Work out the finished part from the listing and answer in its coordinate system (mm). A direction names the side the tool comes from. Round coordinates to 2 decimals unless told otherwise and drop trailing zeros. Write each loop counter-clockwise with the first axis right and the second up, starting at its lowest first coordinate (ties: lowest second). Pieces come first, ordered by that corner, then holes. Notation, with made-up numbers: M 53,-37.5 L 112,-37.5 A25 cw 112,-3.5 Z; hole C 69,4 d8. An arc over 180 degrees is marked long. Answer in a Markdown table with one row per item.
```python
from build123d import *

# Parameters (mm, degrees)
SKETCH1_R           = 6
BOSS_EXTRUDE1_DEPTH = 3
CUT_EXTRUDE4_DEPTH  = 10
BOSS_EXTRUDE2_DEPTH = 5
SKETCH3_R           = 4.5
BOSS_EXTRUDE3_DEPTH = 1
SKETCH4_R           = 3
CUT_EXTRUDE1_DEPTH  = 2
SKETCH5_R           = 1.5
CUT_EXTRUDE2_DEPTH  = 48.699580711
SKETCH6_R           = 1
CUT_EXTRUDE3_DEPTH  = 10
SKETCH8_R           = 1.5
CUT_EXTRUDE5_DEPTH  = 2
SKETCH9_R           = 1
CUT_EXTRUDE6_DEPTH  = 10


with BuildPart() as part:
    # Sketch1 → Boss-Extrude1 (new body)
    with BuildSketch(Plane(origin=(0, 0, 0), x_dir=(1, 0, 0), z_dir=(0, 1, 0))):
        with Locations(Location((0, 0, 0), (0, 0, 270))):
            Circle(SKETCH1_R)
    extrude(amount=BOSS_EXTRUDE1_DEPTH)

    # Sketch7 → Cut-Extrude4 (cut, through all)
    with BuildSketch(Plane.XZ):
        with BuildLine():
            Line((0.7, 3.684087404), (0, 3.05))
            Line((0, 3.05), (-0.7, 3.684087404))
            ThreePointArc((-0.7, 3.684087404), (-0.779668841, 3.668053503), (-0.858971523, 3.650296964))
            Line((-0.858971523, 3.650296964), (-1.240546761, 2.786313646))
            Line((-1.240546761, 2.786313646), (-2.137935164, 3.080865663))
            ThreePointArc((-2.137935164, 3.080865663), (-2.204194696, 3.033813729), (-2.269419066, 2.985337016))
            Line((-2.269419066, 2.985337016), (-2.266591718, 2.040848349))
            Line((-2.266591718, 2.040848349), (-3.206201915, 1.944934261))
            ThreePointArc((-3.206201915, 1.944934261), (-3.247595264, 1.875), (-3.287463436, 1.804185178))
            Line((-3.287463436, 1.804185178), (-2.900722375, 0.942501833))
            Line((-2.900722375, 0.942501833), (-3.720087228, 0.472706055))
            ThreePointArc((-3.720087228, 0.472706055), (-3.729457108, 0.391981737), (-3.737075512, 0.311073332))
            Line((-3.737075512, 0.311073332), (-3.033291781, -0.318811813))
            Line((-3.033291781, -0.318811813), (-3.590735663, -1.081257322))
            ThreePointArc((-3.590735663, -1.081257322), (-3.566461936, -1.158813729), (-3.540513282, -1.235825919))
            Line((-3.540513282, -1.235825919), (-2.641377482, -1.525))
            Line((-2.641377482, -1.525), (-2.840513282, -2.448261485))
            ThreePointArc((-2.840513282, -2.448261485), (-2.786793096, -2.509239774), (-2.73176414, -2.569039642))
            Line((-2.73176414, -2.569039642), (-1.792745019, -2.467501833))
            Line((-1.792745019, -2.467501833), (-1.599140348, -3.391938995))
            ThreePointArc((-1.599140348, -3.391938995), (-1.525262412, -3.425795466), (-1.450668162, -3.458043072))
            Line((-1.450668162, -3.458043072), (-0.634130657, -2.983350182))
            Line((-0.634130657, -2.983350182), (-0.081261521, -3.749119439))
            ThreePointArc((-0.081261521, -3.749119439), (0, -3.75), (0.081261521, -3.749119439))
            Line((0.081261521, -3.749119439), (0.634130657, -2.983350182))
            Line((0.634130657, -2.983350182), (1.450668162, -3.458043072))
            ThreePointArc((1.450668162, -3.458043072), (1.525262412, -3.425795466), (1.599140348, -3.391938995))
            Line((1.599140348, -3.391938995), (1.792745019, -2.467501833))
            Line((1.792745019, -2.467501833), (2.73176414, -2.569039642))
            ThreePointArc((2.73176414, -2.569039642), (2.786793096, -2.509239774), (2.840513282, -2.448261485))
            Line((2.840513282, -2.448261485), (2.641377482, -1.525))
            Line((2.641377482, -1.525), (3.540513282, -1.235825919))
            ThreePointArc((3.540513282, -1.235825919), (3.566461936, -1.158813729), (3.590735663, -1.081257322))
            Line((3.590735663, -1.081257322), (3.033291781, -0.318811813))
            Line((3.033291781, -0.318811813), (3.737075512, 0.311073332))
            ThreePointArc((3.737075512, 0.311073332), (3.729457108, 0.391981737), (3.720087228, 0.472706055))
            Line((3.720087228, 0.472706055), (2.900722375, 0.942501833))
            Line((2.900722375, 0.942501833), (3.287463436, 1.804185178))
            ThreePointArc((3.287463436, 1.804185178), (3.247595264, 1.875), (3.206201915, 1.944934261))
            Line((3.206201915, 1.944934261), (2.266591718, 2.040848349))
            Line((2.266591718, 2.040848349), (2.269419066, 2.985337016))
            ThreePointArc((2.269419066, 2.985337016), (2.204194696, 3.033813729), (2.137935164, 3.080865663))
            Line((2.137935164, 3.080865663), (1.240546761, 2.786313646))
            Line((1.240546761, 2.786313646), (0.858971523, 3.650296964))
            ThreePointArc((0.858971523, 3.650296964), (0.779668841, 3.668053503), (0.7, 3.684087404))
        make_face()
    extrude(amount=-CUT_EXTRUDE4_DEPTH, mode=Mode.SUBTRACT)

    # Sketch2 → Boss-Extrude2 (add)
    with BuildSketch(Plane(origin=(0, 3, 0), x_dir=(1, 0, 0), z_dir=(0, 1, 0))):
        with BuildLine():
            Line((8, 0), (3.5, -43))
            ThreePointArc((3.5, -43), (0, -46.5), (-3.5, -43))
            Line((-3.5, -43), (-8, 0))
            ThreePointArc((-8, 0), (0, 8), (8, 0))
        make_face()
    extrude(amount=BOSS_EXTRUDE2_DEPTH)

    # Sketch3 → Boss-Extrude3 (add)
    with BuildSketch(Plane(origin=(0, 8, 0), x_dir=(1, 0, 0), z_dir=(0, 1, 0))):
        with Locations(Location((0, 0, 0), (0, 0, 270))):
            Circle(SKETCH3_R)
    extrude(amount=BOSS_EXTRUDE3_DEPTH)

    # Sketch4 → Cut-Extrude1 (cut)
    with BuildSketch(Plane(origin=(0, 9, 0), x_dir=(1, 0, 0), z_dir=(0, 1, 0))):
        with Locations(Location((0, 0, 0), (0, 0, 270))):
            Circle(SKETCH4_R)
    extrude(amount=-CUT_EXTRUDE1_DEPTH, mode=Mode.SUBTRACT)

    # Sketch5 → Cut-Extrude2 (cut, through all)
    with BuildSketch(Plane(origin=(0, 7, 0), x_dir=(1, 0, 0), z_dir=(0, 1, 0))):
        with Locations(Location((0, 0, 0), (0, 0, 270))):
            Circle(SKETCH5_R)
    extrude(amount=-CUT_EXTRUDE2_DEPTH, mode=Mode.SUBTRACT)

    # Sketch6 → Cut-Extrude3 (cut)
    with BuildSketch(Plane(origin=(0, 8, 0), x_dir=(1, 0, 0), z_dir=(0, 1, 0))):
        with Locations(Location((0, -13, 0), (0, 0, 270))):
            Circle(SKETCH6_R)
        with Locations(Location((0, -18, 0), (0, 0, 270))):
            Circle(SKETCH6_R)
        with Locations(Location((0, -23, 0), (0, 0, 270))):
            Circle(SKETCH6_R)
        with Locations(Location((0, -28, 0), (0, 0, 270))):
            Circle(SKETCH6_R)
        with Locations(Location((0, -33, 0), (0, 0, 270))):
            Circle(SKETCH6_R)
        with Locations(Location((0, -38, 0), (0, 0, 270))):
            Circle(SKETCH6_R)
        with Locations(Location((0, -43, 0), (0, 0, 270))):
            Circle(SKETCH6_R)
    extrude(amount=-CUT_EXTRUDE3_DEPTH, mode=Mode.SUBTRACT)

    # Sketch8 → Cut-Extrude5 (cut)
    with BuildSketch(Plane.XZ.offset(-3)):
        with BuildLine():
            Line((-0.858971523, 3.650296964), (-1.240546761, 2.786313646))
            Line((-1.240546761, 2.786313646), (-2.137935164, 3.080865663))
            ThreePointArc((-2.137935164, 3.080865663), (-2.204194696, 3.033813729), (-2.269419066, 2.985337016))
            Line((-2.269419066, 2.985337016), (-2.266591718, 2.040848349))
            Line((-2.266591718, 2.040848349), (-3.206201915, 1.944934261))
            ThreePointArc((-3.206201915, 1.944934261), (-3.247595264, 1.875), (-3.287463436, 1.804185178))
            Line((-3.287463436, 1.804185178), (-2.900722375, 0.942501833))
            Line((-2.900722375, 0.942501833), (-3.720087228, 0.472706055))
            ThreePointArc((-3.720087228, 0.472706055), (-3.729457108, 0.391981737), (-3.737075512, 0.311073332))
            Line((-3.737075512, 0.311073332), (-3.033291781, -0.318811813))
            Line((-3.033291781, -0.318811813), (-3.590735663, -1.081257322))
            ThreePointArc((-3.590735663, -1.081257322), (-3.566461936, -1.158813729), (-3.540513282, -1.235825919))
            Line((-3.540513282, -1.235825919), (-2.641377482, -1.525))
            Line((-2.641377482, -1.525), (-2.840513282, -2.448261485))
            ThreePointArc((-2.840513282, -2.448261485), (-2.786793096, -2.509239774), (-2.73176414, -2.569039642))
            Line((-2.73176414, -2.569039642), (-1.792745019, -2.467501833))
            Line((-1.792745019, -2.467501833), (-1.599140348, -3.391938995))
            ThreePointArc((-1.599140348, -3.391938995), (-1.525262412, -3.425795466), (-1.450668162, -3.458043072))
            Line((-1.450668162, -3.458043072), (-0.634130657, -2.983350182))
            Line((-0.634130657, -2.983350182), (-0.081261521, -3.749119439))
            ThreePointArc((-0.081261521, -3.749119439), (0, -3.75), (0.081261521, -3.749119439))
            Line((0.081261521, -3.749119439), (0.634130657, -2.983350182))
            Line((0.634130657, -2.983350182), (1.450668162, -3.458043072))
            ThreePointArc((1.450668162, -3.458043072), (1.525262412, -3.425795466), (1.599140348, -3.391938995))
            Line((1.599140348, -3.391938995), (1.792745019, -2.467501833))
            Line((1.792745019, -2.467501833), (2.73176414, -2.569039642))
            ThreePointArc((2.73176414, -2.569039642), (2.786793096, -2.509239774), (2.840513282, -2.448261485))
            Line((2.840513282, -2.448261485), (2.641377482, -1.525))
            Line((2.641377482, -1.525), (3.540513282, -1.235825919))
            ThreePointArc((3.540513282, -1.235825919), (3.566461936, -1.158813729), (3.590735663, -1.081257322))
            Line((3.590735663, -1.081257322), (3.033291781, -0.318811813))
            Line((3.033291781, -0.318811813), (3.737075512, 0.311073332))
            ThreePointArc((3.737075512, 0.311073332), (3.729457108, 0.391981737), (3.720087228, 0.472706055))
            Line((3.720087228, 0.472706055), (2.900722375, 0.942501833))
            Line((2.900722375, 0.942501833), (3.287463436, 1.804185178))
            ThreePointArc((3.287463436, 1.804185178), (3.247595264, 1.875), (3.206201915, 1.944934261))
            Line((3.206201915, 1.944934261), (2.266591718, 2.040848349))
            Line((2.266591718, 2.040848349), (2.269419066, 2.985337016))
            ThreePointArc((2.269419066, 2.985337016), (2.204194696, 3.033813729), (2.137935164, 3.080865663))
            Line((2.137935164, 3.080865663), (1.240546761, 2.786313646))
            Line((1.240546761, 2.786313646), (0.858971523, 3.650296964))
            ThreePointArc((0.858971523, 3.650296964), (0.779668841, 3.668053503), (0.7, 3.684087404))
            Line((0.7, 3.684087404), (0, 3.05))
            Line((0, 3.05), (-0.7, 3.684087404))
            ThreePointArc((-0.7, 3.684087404), (-0.779668841, 3.668053503), (-0.858971523, 3.650296964))
        make_face()
        with Locations(Location((0, 0, 0), (0, 0, 90))):
            Circle(SKETCH8_R, mode=Mode.SUBTRACT)
    extrude(amount=-CUT_EXTRUDE5_DEPTH, mode=Mode.SUBTRACT)

    # Sketch9 → Cut-Extrude6 (cut)
    with BuildSketch(Plane(origin=(0, 8, 0), x_dir=(1, 0, 0), z_dir=(0, 1, 0))):
        with BuildLine():
            ThreePointArc((-0.999557496, -32.970254191), (-3.566749104, -31.602893663), (-4.959923611, -29.049618831))
            Line((-4.959923611, -29.049618831), (-3.5, -43))
            ThreePointArc((-3.5, -43), (0, -46.5), (3.5, -43))
            Line((3.5, -43), (4.959923611, -29.049618831))
            ThreePointArc((4.959923611, -29.049618831), (3.566749104, -31.602893663), (0.999557496, -32.970254191))
            ThreePointArc((0.999557496, -32.970254191), (0.999889368, -32.98512545), (1, -33))
            ThreePointArc((1, -33), (-0.01487455, -33.999889368), (-0.999557496, -32.970254191))
        make_face()
        with Locations((0, -43)):
            Circle(SKETCH9_R, mode=Mode.SUBTRACT)
        with Locations((0, -38)):
            Circle(SKETCH9_R, mode=Mode.SUBTRACT)
    extrude(amount=-CUT_EXTRUDE6_DEPTH, mode=Mode.SUBTRACT)


solid = part.part
```
1. A tool of negligible diameter and unlimited length cuts with its end or side. For faces 1 (the flat face through (-1.3, 7, 1.3)), 2 (the flat face through (-2.73, 2.465, 1.994)), 3 (the cylindrical face through (0, 6, 14)), from which of +Z, -Z, +X, -X, +Y, -Y can it reach the whole face along a straight path? Write none if from no direction.
Calculated:
| item | result |
|---|---|
| face 1 | +Y |
| face 2 | -Y |
| face 3 | +Y, -Y |
2. Determine the mould class of faces 4 (the cylindrical face through (-3.54, 5.54, 31.63)), 5 (the flat face through (-3, 9, 1)), 6 (the flat face through (1.695, 2.465, -2.936)) for opening direction X: released by +X, released by -X, zero draft, split by the parting line, or undercut.
Calculated:
| item | result |
|---|---|
| face 4 | released by -X |
| face 5 | zero draft |
| face 6 | undercut |
3. The part is cut by section B-B (z = 23). Determine the outline of the cut face in (x, y), plus the area to 3 significant figures.
Calculated:
| item | result |
|---|---|
| outline | M -5.59,3 L -1,3 L -1,8 L -5.59,8 Z; M 1,3 L 5.59,3 L 5.59,8 L 1,8 Z |
| area | 45.9 mm² |
4. Consider line 1 along X through (y, z) = (6.55, 0); line 2 along Y through (x, z) = (0.25, 31); line 3 along Y through (x, z) = (-1.5, 4.5). Determine where each line is inside the solid, lowest interval first. Write a range as from..to.
Calculated:
| item | result |
|---|---|
| line 1 | x = -8..-1.5, 1.5..8 |
| line 2 | y = 3..8 |
| line 3 | y = 0..8 |
5. The part is cut by section A-A (z = 13). Determine the outline of the cut face in (x, y), plus the area to 3 significant figures.
Calculated:
| item | result |
|---|---|
| outline | M -6.64,3 L -1,3 L -1,8 L -6.64,8 Z; M 1,3 L 6.64,3 L 6.64,8 L 1,8 Z |
| area | 56.4 mm² |
6. Given pin 1 (4 mm diameter, centred on x = 6, y = 8, fed in from -Z); pin 2 (4 mm diameter, centred on x = 0, y = 6, fed in from +Z); pin 3 (5 mm diameter, centred on x = -2, z = 13, fed in from -Y); pin 4 (1.8 mm diameter, centred on x = 0, z = 0, fed in from -Y), each flat-ended and moving along its own axis, determine where each tip first touches the part or whether it passes through.
Calculated:
| item | result |
|---|---|
| pin 1 | stops at z = -6.93 |
| pin 2 | stops at z = 32.97 |
| pin 3 | stops at y = 3 |
| pin 4 | passes through |
7. The part is cut by section C-C (z = 6.5). Determine the outline of the cut face in (x, y).
Calculated:
| item | result |
|---|---|
| outline | M -7.32,3 L 7.32,3 L 7.32,8 L -7.32,8 Z |
